Part model, mm, in its own coordinate system. A direction names the side the tool comes from. Give positions to 0.01 mm unless a question says otherwise; leave off trailing zeros. Loops run counter-clockwise (first coordinate to the right, second up) from the corner with the lowest first, then second, coordinate; pieces in that order, holes last. Notation, with made-up numbers: (20, 0.25) -> (57, 0.25) arc R29 ccw to (57, 37.25) -> close; hole circle Ø11 at (68, 74). An arc over 180 degrees is marked (long way). Write item = value, one per line.
from build123d import *

# Parameters (mm, degrees)
SKETCH1_W           = 190.5
SKETCH1_H           = 190.5
BOSS_EXTRUDE1_DEPTH = 9.525
SKETCH2_W           = 38.1
SKETCH2_H           = 9.525
CUT_EXTRUDE1_DEPTH  = 9.525
SKETCH3_W           = 38.1
SKETCH3_H           = 9.525
CUT_EXTRUDE2_DEPTH  = 9.525
SKETCH4_W           = 9.525
SKETCH4_H           = 28.575
CUT_EXTRUDE3_DEPTH  = 9.525
SKETCH5_W           = 9.525
SKETCH5_H           = 38.1
CUT_EXTRUDE4_DEPTH  = 9.525
SKETCH6_W           = 9.525
SKETCH6_H           = 28.575
CUT_EXTRUDE5_DEPTH  = 9.525
SKETCH7_W           = 38.1
SKETCH7_H           = 9.525
CUT_EXTRUDE6_DEPTH  = 9.525
SKETCH8_W           = 38.1
SKETCH8_H           = 9.525
CUT_EXTRUDE7_DEPTH  = 9.525
SKETCH9_W           = 9.525
SKETCH9_H           = 28.575
CUT_EXTRUDE8_DEPTH  = 38.1
SKETCH10_W          = 9.525
SKETCH10_H          = 38.1
CUT_EXTRUDE9_DEPTH  = 9.525
SKETCH11_W          = 9.525
SKETCH11_H          = 28.575
CUT_EXTRUDE10_DEPTH = 9.525
SKETCH12_W          = 25.4
SKETCH12_H          = 9.525
CUT_EXTRUDE11_DEPTH = 12.7


with BuildPart() as part:
    # Sketch1 → Boss-Extrude1 (new body)
    with BuildSketch(Plane(origin=(0, 0, 0), x_dir=(1, 0, 0), z_dir=(0, 1, 0))):
        with Locations((61.628840928, 48.799714441)):
            Rectangle(SKETCH1_W, SKETCH1_H)
    extrude(amount=BOSS_EXTRUDE1_DEPTH)

    # Sketch2 → Cut-Extrude1 (cut)
    with BuildSketch(Plane(origin=(0, 9.525, 0), x_dir=(1, 0, 0), z_dir=(0, 1, 0))):
        with Locations((99.728840928, -41.687785559)):
            Rectangle(SKETCH2_W, SKETCH2_H)
    extrude(amount=-CUT_EXTRUDE1_DEPTH, mode=Mode.SUBTRACT)

    # Sketch3 → Cut-Extrude2 (cut)
    with BuildSketch(Plane(origin=(0, 9.525, 0), x_dir=(1, 0, 0), z_dir=(0, 1, 0))):
        with Locations((23.528840928, -41.687785559)):
            Rectangle(SKETCH3_W, SKETCH3_H)
    extrude(amount=-CUT_EXTRUDE2_DEPTH, mode=Mode.SUBTRACT)

    # Sketch4 → Cut-Extrude3 (cut)
    with BuildSketch(Plane(origin=(0, 9.525, 0), x_dir=(1, 0, 0), z_dir=(0, 1, 0))):
        with Locations((152.116340928, -22.637785559)):
            Rectangle(SKETCH4_W, SKETCH4_H)
    extrude(amount=-CUT_EXTRUDE3_DEPTH, mode=Mode.SUBTRACT)

    # Sketch5 → Cut-Extrude4 (cut)
    with BuildSketch(Plane(origin=(0, 9.525, 0), x_dir=(1, 0, 0), z_dir=(0, 1, 0))):
        with Locations((152.116340928, 48.799714441)):
            Rectangle(SKETCH5_W, SKETCH5_H)
    extrude(amount=-CUT_EXTRUDE4_DEPTH, mode=Mode.SUBTRACT)

    # Sketch6 → Cut-Extrude5 (cut)
    with BuildSketch(Plane(origin=(0, 9.525, 0), x_dir=(1, 0, 0), z_dir=(0, 1, 0))):
        with Locations((152.116340928, 120.237214441)):
            Rectangle(SKETCH6_W, SKETCH6_H)
    extrude(amount=-CUT_EXTRUDE5_DEPTH, mode=Mode.SUBTRACT)

    # Sketch7 → Cut-Extrude6 (cut)
    with BuildSketch(Plane(origin=(0, 9.525, 0), x_dir=(1, 0, 0), z_dir=(0, 1, 0))):
        with Locations((99.728840928, 139.287214441)):
            Rectangle(SKETCH7_W, SKETCH7_H)
    extrude(amount=-CUT_EXTRUDE6_DEPTH, mode=Mode.SUBTRACT)

    # Sketch8 → Cut-Extrude7 (cut)
    with BuildSketch(Plane(origin=(0, 9.525, 0), x_dir=(1, 0, 0), z_dir=(0, 1, 0))):
        with Locations((23.528840928, 139.287214441)):
            Rectangle(SKETCH8_W, SKETCH8_H)
    extrude(amount=-CUT_EXTRUDE7_DEPTH, mode=Mode.SUBTRACT)

    # Sketch9 → Cut-Extrude8 (cut)
    with BuildSketch(Plane(origin=(0, 9.525, 0), x_dir=(1, 0, 0), z_dir=(0, 1, 0))):
        with Locations((-28.858659072, 120.237214441)):
            Rectangle(SKETCH9_W, SKETCH9_H)
    extrude(amount=-CUT_EXTRUDE8_DEPTH, mode=Mode.SUBTRACT)

    # Sketch10 → Cut-Extrude9 (cut)
    with BuildSketch(Plane(origin=(0, 9.525, 0), x_dir=(1, 0, 0), z_dir=(0, 1, 0))):
        with Locations((-28.858659072, 48.799714441)):
            Rectangle(SKETCH10_W, SKETCH10_H)
    extrude(amount=-CUT_EXTRUDE9_DEPTH, mode=Mode.SUBTRACT)

    # Sketch11 → Cut-Extrude10 (cut)
    with BuildSketch(Plane(origin=(0, 9.525, 0), x_dir=(1, 0, 0), z_dir=(0, 1, 0))):
        with Locations((-28.858659072, -22.637785559)):
            Rectangle(SKETCH11_W, SKETCH11_H)
    extrude(amount=-CUT_EXTRUDE10_DEPTH, mode=Mode.SUBTRACT)

    # Sketch12 → Cut-Extrude11 (cut)
    with BuildSketch(Plane(origin=(0, 9.525, 0), x_dir=(1, 0, 0), z_dir=(0, 1, 0))):
        with Locations((20.353840928, 98.012214441)):
            Rectangle(SKETCH12_W, SKETCH12_H)
        with Locations((102.903840928, 98.012214441)):
            Rectangle(SKETCH12_W, SKETCH12_H)
    extrude(amount=-CUT_EXTRUDE11_DEPTH, mode=Mode.SUBTRACT)


solid = part.part
1) Slice it at C-C, the plane z = 15.5. List the corners of the cut face in (x, y) (3 decimals).
Resolved:
outline = (-24.096, 0) -> (147.354, 0) -> (147.354, 9.525) -> (-24.096, 9.525) -> close
2) Which spindle directions (+Z, -Z, +X, -X, +Y, -Y) get a long thin tool onto all of the face, cutting with end or side? Do faces 1 (the face through (152, 5, -105.95)), 2 (the face through (80.679, 5, 42)), 3 (the face through (-29, 5, -67.85)), 4 (the face through (115.604, 5, -98)). Say none if no direction does.
Resolved:
face_1 = +X, +Y, -Y
face_2 = +Z, +Y, -Y
face_3 = -X, +Y, -Y
face_4 = +Y, -Y
3) Pull direction X, two halves, no side cores. Call faces 5 (the face through (-33.621, 5, -87)), 6 (the face through (80.679, 5, -139)), 7 (the face through (-15, 5, 46.45)), 8 (the face through (23, 5, 36.925)): pulls with the +X half, pulls with the -X half, needs draft (parallel to the pull), parting line crosses it, or undercut.
Resolved:
face_5 = pulls with the -X half
face_6 = undercut
face_7 = needs draft
face_8 = undercut
4) Drill centre lines: line 1 along Z through (x, y) = (30, 3.5); line 2 along Z through (x, y) = (5, 6); line 3 along X through (y, z) = (8.5, -129). Where is each one in solid material? Low to high. Write a range as [from, to].
Resolved:
line_1 = [-134.52, -102.77], [-93.25, 36.93]
line_2 = [-134.52, 36.93]
line_3 = [-24.1, 147.35]
5) Drop flat-ended pins along their axis: P1, Ø4, axis at x = 89.5, y = 7, coming from the -Z side; P2, Ø5, axis at x = 14.5, y = 4, coming from the +Z side; P3, Ø10, axis at x = 99, z = -91.5, coming from the -Y side; P4, Ø3, axis at y = 3, z = -116, coming from the -X side. Give the stop position or say it passes through.
Resolved:
P1 = -134.52
P2 = 36.93
P3 = 0
P4 = -24.1
6) Slice it at B-B, the plane y = 5. Count the separate pieces of the cut face and the enclosed holes in it, and give its area (3 significant figures).
Resolved:
separate_pieces = 1
enclosed_holes = 2
area = 32,500 mm²
7) Slice it at A-A, the plane x = 10. List the corners of the cut face in (y, z) (3 decimals), and give its area (3 significant figures).
Resolved:
outline = (0, -134.525) -> (9.525, -134.525) -> (9.525, -102.775) -> (0, -102.775) -> close; (0, -93.25) -> (9.525, -93.25) -> (9.525, 36.925) -> (0, 36.925) -> close
area = 1,540 mm²
